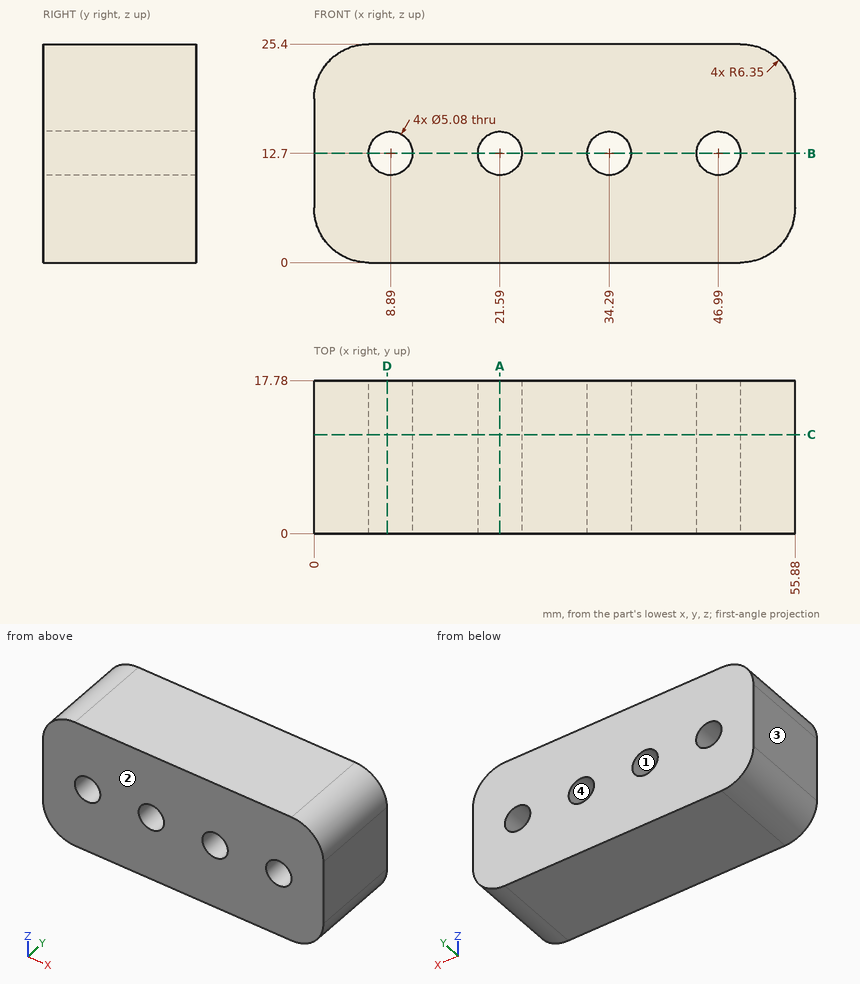
Here's the drawing with two shaded views (mm, measured from the low corner). I have some questions. Give positions to 0.01 mm unless a question says otherwise; leave off trailing zeros. Order: outer loops, then holes, each group sorted by start corner. A loop starts at its lowest first (then second) coordinate and runs counter-clockwise, first axis right, second up. Notation, with made-up numbers: M -32,80.25 L -1,80.25 A21 ccw -1,89.25 Z; hole C 20,-12.5 d3. An arc over 180 degrees is marked long. One line per question, with ' | ' between items.
Item 1: Suppose I cut it at C-C, the plane y = 11.5. Write out the boundary of the cut face in (x, z), then the cut area to 3 significant figures.
Answer block:
outline: M 0,6.35 A6.35 ccw 6.35,0 L 49.53,0 A6.35 ccw 55.88,6.35 L 55.88,19.05 A6.35 ccw 49.53,25.4 L 6.35,25.4 A6.35 ccw 0,19.05 Z; hole C 8.89,12.7 d5.08; hole C 21.59,12.7 d5.08; hole C 34.29,12.7 d5.08; hole C 46.99,12.7 d5.08 | area: 1,300 mm2
Item 2: We'd pull the mould along X, two halves only. Please class the marked faces 1, 2, 3 and 4: released by +X, released by -X, zero draft, split by the parting line, or undercut.
Answer block:
face 1: undercut | face 2: zero draft | face 3: released by -X | face 4: undercut
Item 3: Suppose I cut it at A-A, the plane x = 21.59. Write out the boundary of the cut face in (y, z), then the cut area to 3 significant figures.
Answer block:
outline: M 0,0 L 17.78,0 L 17.78,10.16 L 0,10.16 Z; M 0,15.24 L 17.78,15.24 L 17.78,25.4 L 0,25.4 Z | area: 361 mm2
Item 4: Suppose I cut it at D-D, the plane x = 8.5. Write out the boundary of the cut face in (y, z), then the cut area to 3 significant figures.
Answer block:
outline: M 0,0 L 17.78,0 L 17.78,10.19 L 0,10.19 Z; M 0,15.21 L 17.78,15.21 L 17.78,25.4 L 0,25.4 Z | area: 362 mm2
Item 5: Please list where these lines run through material, in increasing order: L1, parallel to Z at x = 34.29, y = 6.5; L2, parallel to X at y = 14.75, z = 13.75; L3, parallel to Z at x = 35, y = 4.25.
Answer block:
L1: z = 0 to 10.16, 15.24 to 25.4 | L2: x = 0 to 6.58, 11.2 to 19.28, 23.9 to 31.98, 36.6 to 44.68, 49.3 to 55.88 | L3: z = 0 to 10.26, 15.14 to 25.4
Item 6: Suppose I cut it at B-B, the plane z = 12.7. Write out the boundary of the cut face in (x, y).
Answer block:
outline: M 0,0 L 6.35,0 L 6.35,17.78 L 0,17.78 Z; M 11.43,0 L 19.05,0 L 19.05,17.78 L 11.43,17.78 Z; M 24.13,0 L 31.75,0 L 31.75,17.78 L 24.13,17.78 Z; M 36.83,0 L 44.45,0 L 44.45,17.78 L 36.83,17.78 Z; M 49.53,0 L 55.88,0 L 55.88,17.78 L 49.53,17.78 Z
